Design review of the part built by this model. Coordinates are the model's own, in mm. Face numbers are marked on the shaded views. A direction names the side the tool comes from. Coordinates: 2 decimals unless noted, no trailing zeros. Write each loop counter-clockwise with the first axis right and the second up, starting at its lowest first coordinate (ties: lowest second). Pieces come first, ordered by that corner, then holes. Notation, with made-up numbers: M -2.5,-32.5 L 17.5,-32.5 A25 cw 17.5,-0.5 Z; hole C 12,6 d4. An arc over 180 degrees is marked long. One line per question, with ' | ' between items.
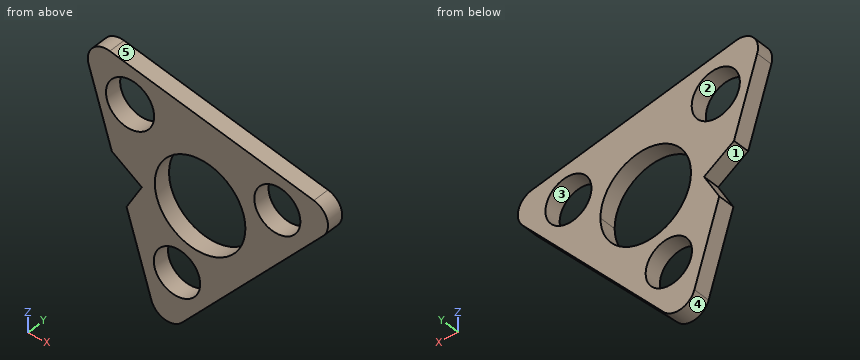
from build123d import *

# Parameters (mm, degrees)
F0_R     = 6.499611
F0_R_2   = 6.748497
F0_R_3   = 6.451892
F1_DEPTH = 4.826
F2_R     = 5.08


with BuildPart() as f1:
    # F0 (on Front) → F1 (new body)
    with BuildSketch(Plane.XZ):
        Polygon((-9.602852, -191.570323), (0, -222.072359), (20.980663, -199.195719), (51.504101, -165.913944), (-22.882563, -149.389291), (-13.740194, -178.42867), (-5.334256, -184.135315), align=None)
        with Locations((4.538138, -202.582002)):
            Circle(F0_R, mode=Mode.SUBTRACT)
        with BuildLine():
            ThreePointArc((23.719741, -181.157266), (23.015442, -185.327775), (20.980663, -189.035719))
            ThreePointArc((20.980663, -189.035719), (-0.975961, -176.986757), (23.719741, -181.157266))
        make_face(mode=Mode.SUBTRACT)
        with Locations((-8.626509, -163.088083)):
            Circle(F0_R_2, mode=Mode.SUBTRACT)
        with Locations((32.683235, -171.713188)):
            Circle(F0_R_3, mode=Mode.SUBTRACT)
    extrude(amount=F1_DEPTH)

    # F2
    f2_edges = [f1.edges().sort_by_distance(p)[0] for p in [
        (0, -2.413, -222.072359),
        (51.504101, -2.413, -165.913944),
        (-22.882563, -2.413, -149.389291),
    ]]
    fillet(f2_edges, radius=F2_R)


solid = f1.part
1. Take a section at C-C (x = 9.5). Write out the cut boundary in (y, z).
Answer sheet:
outline: M -4.83,-211.71 L 0,-211.71 L 0,-206.78 L -4.83,-206.78 Z; M -4.83,-198.38 L 0,-198.38 L 0,-193.77 L -4.83,-193.77 Z; M -4.83,-168.55 L 0,-168.55 L 0,-156.58 L -4.83,-156.58 Z
2. Take a section at D-D (y = -1.15). Write out the cut boundary in (x, z).
Answer sheet:
outline: M -20.24,-157.78 L -13.74,-178.43 L -5.33,-184.14 L -9.6,-191.57 L -2.64,-213.68 A5.08 ccw 5.95,-215.59 L 45.56,-172.4 A5.08 ccw 42.91,-164.01 L -14.29,-151.3 A5.08 ccw Z; hole C -8.63,-163.09 d13.5; hole C 4.54,-202.58 d13; hole M 20.98,-189.04 A12.7 ccw 23.72,-181.16 A12.7 ccw long Z; hole C 32.68,-171.71 d12.9
3. Insertion check: pin 1 Ø17 at (x, z) = (4.54, -202.58) entering from -Y; pin 2 Ø8 at (x, z) = (-8.63, -163.09) entering from -Y; pin 3 Ø1 at (x, y) = (4, -3.5) entering from +Z; pin 4 Ø1 at (x, y) = (-10.5, -2.5) entering from -Z. Each pin has a flat end and moves straight along its axis. Give the tip position at first contact, or say it passes through.
Answer sheet:
pin 1: y = -4.83 | pin 2: through | pin 3: z = -155.25 | pin 4: z = -180.97
4. Tool access review of the marked faces 1 and 2: name each direction out of +Z, -Z, +X, -X, +Y, -Y from which nothing blocks a thin tool from reaching the whole face with its end or side.
Answer sheet:
face 1: -X, +Y, -Y | face 2: +Y, -Y
5. Take a section at B-B (z = -190.5). Write out the cut boundary in (x, y).
Answer sheet:
outline: M -8.99,-4.83 L 2.42,-4.83 L 2.42,0 L -8.99,0 Z; M 19.62,-4.83 L 28.96,-4.83 L 28.96,0 L 19.62,0 Z
6. Take a section at A-A (x = 35). Write out the cut boundary in (y, z), then the cut area to 3 significant figures.
Answer sheet:
outline: M -4.83,-183.91 L 0,-183.91 L 0,-177.73 L -4.83,-177.73 Z; M -4.83,-165.69 L 0,-165.69 L 0,-162.25 L -4.83,-162.25 Z | area: 46.4 mm^2
7. To check wall thickness, follow line 1 along X through (y, z) = (-3.2, -167.5); line 2 along X through (y, z) = (-1.2, -166.5); line 3 along Z through (x, y) = (10, -1.25). State the ranges of each line that lie inside material, in increasing order. Write a range as [from, to].
Answer sheet:
line 1: [-17.18, -13.73], [-3.52, 27.8], [37.57, 46.68] | line 2: [-17.5, -14.45], [-2.8, 28.88], [36.48, 46.25] | line 3: [-211.17, -206.11], [-199.06, -193.82], [-168.5, -156.69]
8. Draft analysis for pull direction Z (two halves, no side actions). For the marked faces 3, 4 and 5, state which applies: pulls with the +Z half, pulls with the -Z half, needs draft (parallel to the pull), parting line crosses it, or undercut.
Answer sheet:
face 3: undercut | face 4: pulls with the -Z half | face 5: pulls with the +Z half
